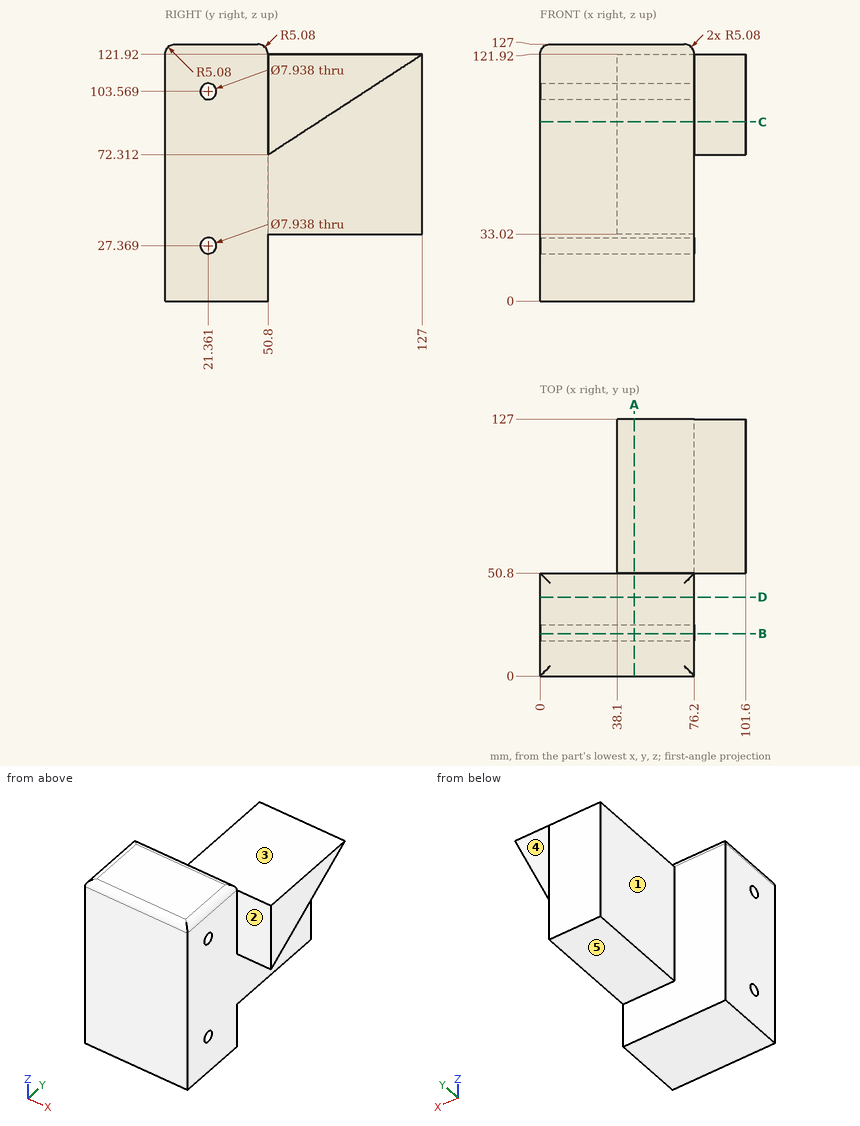
Geometry check sheet. Reference: drawing and pictorial views, mm from the part's lowest x, y, z. A direction names the side the tool comes from. Round coordinates to 2 decimals unless told otherwise and drop trailing zeros. Loops run counter-clockwise (first coordinate to the right, second up) from the corner with the lowest first, then second, coordinate; pieces in that order, holes last. Notation, with made-up numbers: M 26,70 L 49,70 A14 cw 49,79 Z; hole C -28,-8 d4. An arc over 180 degrees is marked long. Return JSON: item names as keys, results as strings. Group by question number.
(1) Section check A-A, the plane x = 46.5. Enter the section's corners in (y, z).
(2) Section check C-C, the plane z = 88.5. Enter the section's corners in (x, y) (1 decimal), and give its area (3 significant figures).
(3) Section check D-D, the plane y = 39. Enter the section's corners in (x, z).
(4) Scan lines: line 1 along X through (y, z) = (89, 70.5); line 2 along Y through (x, z) = (34, 121.5); line 3 along Y through (x, z) = (7, 26) (1 decimal). Record each from-to range of solid material in increasing order. Write a range as [from, to].
(5) Go/stop test with flat-tipped pins: pin 1 (5 mm diameter, centred on y = 21.36, z = 103.57, fed in from -X); pin 2 (1 mm diameter, centred on x = 18, z = 24.5, fed in from +Y); pin 3 (6 mm diameter, centred on y = 29.5, z = 80.5, fed in from +X); pin 4 (6 mm diameter, centred on x = 50.5, y = 113, fed in from -Z). Record where each tip stops, or that it passes through.
(6) Set-up check for the marked faces 1, 2, 3, 4 and 5: record each of +Z, -Z, +X, -X, +Y, -Y from which the full face is reachable in a straight line by a thin tool's end or side.
(7) Section check B-B, the plane y = 21. Enter the section's corners in (x, z), and give its area (3 significant figures).
Data:
{
 "1": {"outline": "M 0,0 L 50.8,0 L 50.8,33.02 L 127,33.02 L 127,121.92 L 50.8,121.92 A5.08 ccw 45.72,127 L 5.08,127 A5.08 ccw 0,121.92 Z; hole C 21.36,27.37 d7.94; hole C 21.36,103.57 d7.94"},
 "2": {"outline": "M 0,0 L 76.2,0 L 76.2,50.8 L 101.6,50.8 L 101.6,75.7 L 76.2,75.7 L 76.2,127 L 38.1,127 L 38.1,50.8 L 0,50.8 Z", "area": "7,410 mm²"},
 "3": {"outline": "M 0,0 L 76.2,0 L 76.2,121.92 A5.08 ccw 71.12,127 L 5.08,127 A5.08 ccw 0,121.92 Z"},
 "4": {"line 1": "[38.1, 76.2]", "line 2": "[0, 50.8]", "line 3": "[0, 17.6], [25.1, 50.8]"},
 "5": {"pin 1": "through", "pin 2": "y = 50.8", "pin 3": "x = 76.2", "pin 4": "z = 33.02"},
 "6": {"face 1": "+Z, -Z, -X, +Y", "face 2": "+Z, -Z, +X, -Y", "face 3": "+Z, +X, -X, +Y", "face 4": "-Z, +X, +Y", "face 5": "-Z, +X, -X, +Y"},
 "7": {"outline": "M 0,0 L 76.2,0 L 76.2,23.42 L 0,23.42 Z; M 0,31.32 L 76.2,31.32 L 76.2,99.62 L 0,99.62 Z; M 0,107.52 L 76.2,107.52 L 76.2,121.92 A5.08 ccw 71.12,127 L 5.08,127 A5.08 ccw 0,121.92 Z", "area": "8,460 mm²"}
}
